CAD build for the part. Positions are in the model's coordinates, mm. A direction names the side the tool comes from. Round coordinates to 2 decimals unless told otherwise and drop trailing zeros. Order: outer loops, then holes, each group sorted by start corner. A loop starts at its lowest first (then second) coordinate and runs counter-clockwise, first axis right, second up. Notation, with made-up numbers: M 89,28.5 L 145,28.5 A17 cw 145,43.5 Z; hole C 27,73 d3. An arc over 180 degrees is marked long. Answer as a JSON object with one key per item and string values. Group by question number.
```python
from build123d import *

# Parameters (mm, degrees)
BOSS_EXTRUDE1_DEPTH = 36
FILLET2_R           = 8
SKETCH4_R           = 4
CUT_EXTRUDE2_DEPTH  = 32.38102997
SKETCH3_R           = 3
CUT_EXTRUDE3_DEPTH  = 12


with BuildPart() as part:
    # Sketch2 → Boss-Extrude1 (new body, symmetric)
    with BuildSketch(Plane(origin=(0, 0, 0), x_dir=(0, 0, -1), z_dir=(1, 0, 0))):
        Polygon((37.235479123, 0), (37.235479123, 12), (-34.764520877, 32.645667775), (-34.764520877, 0), align=None)
    extrude(amount=BOSS_EXTRUDE1_DEPTH, both=True)

    # Fillet2
    fillet2_edges = [part.edges().sort_by_distance(p)[0] for p in [
        (36, 6, -37.235479123),
        (-36, 6, -37.235479123),
        (-36, 16.322833887, 34.764520877),
        (36, 16.322833887, 34.764520877),
    ]]
    fillet(fillet2_edges, radius=FILLET2_R)

    # Sketch4 → Cut-Extrude2 (cut, through all)
    with BuildSketch(Plane(origin=(0, 20.954187427, -6.008516557), x_dir=(1, 0, 0), z_dir=(0, 0.961261696, -0.275637356))):
        with Locations((-23, 19.485391541)):
            Circle(SKETCH4_R)
    extrude(amount=-CUT_EXTRUDE2_DEPTH, mode=Mode.SUBTRACT)

    # Sketch3 → Cut-Extrude3 (cut)
    with BuildSketch(Plane(origin=(0, 20.954187427, -6.008516557), x_dir=(1, 0, 0), z_dir=(0, 0.961261696, -0.275637356))):
        with Locations((-20, -28.416167841)):
            Circle(SKETCH3_R)
        with Locations((-6, -28.416167841)):
            Circle(SKETCH3_R)
        with Locations((8, -28.416167841)):
            Circle(SKETCH3_R)
        with Locations((22, -28.416167841)):
            Circle(SKETCH3_R)
        with Locations((22, -14.416167841)):
            Circle(SKETCH3_R)
        with Locations((22, -0.416167841)):
            Circle(SKETCH3_R)
        with Locations((22, 13.583832159)):
            Circle(SKETCH3_R)
    extrude(amount=-CUT_EXTRUDE3_DEPTH, mode=Mode.SUBTRACT)


solid = part.part
```
Item 1: Drill centre lines: line 1 (X direction, y = 16.5, z = -4.5); line 2 (X direction, y = 2.5, z = -24); line 3 (Z direction, x = -25.5, y = 8). Where is each one in solid material? Low to high. Write a range as [from, to].
Item 2: Two-plate mould, pull along Y, no slides. Class faces 1 (the face through (0.5, 22.18, -1.74)), 2 (the face through (-33.594, 16.094, 32.483)), 3 (the face through (19, 19.2, 9.4)): +Y half, -Y half, draft (parallel to the pull), parting line (faces both ways), or undercut.
Item 3: Cut at A-A, the plane x = -8. Give the cut face in (y, z).
Item 4: Cut at B-B, the plane z = 29. Give the cut face in (x, y), and give its area (3 significant figures).
Item 5: Flat gauge pins, fed straight in: pin 1 Ø5 at (y, z) = (15.5, -29.5) entering from -X; pin 2 Ø10 at (x, z) = (-22.5, -27) entering from +Y. Where does each tip first touch, or does it go through?
Item 6: Cut at C-C, the plane x = 12. Give the cut face in (y, z).
Item 7: 3-axis set-ups, long thin cutter, end or side, ignore diameter. For faces 4 (the face through (7.96, 17.24, 24.57)), 5 (the face through (1, 0, -1)): which of +Z, -Z, +X, -X, +Y, -Y reach the whole face in a straight line?
Response values:
{
 "1": {"line 1": "[-36, 19.01], [24.99, 36]", "line 2": "[-36, -25.76], [-20.24, 36]", "line 3": "[-37.24, -25.81], [-19.32, 34.76]"},
 "2": {"face 1": "+Y half", "face 2": "draft", "face 3": "undercut"},
 "3": {"outline": "M 0,-37.24 L 12,-37.24 L 28.17,19.16 L 16.64,22.47 L 17.87,26.76 L 29.4,23.46 L 32.65,34.76 L 0,34.76 Z"},
 "4": {"outline": "M -35.68,0 L 35.68,0 L 35.68,30.99 L -35.68,30.99 Z", "area": "2,210 mm^2"},
 "5": {"pin 1": "x = -36", "pin 2": "y = 16.06"},
 "6": {"outline": "M 0,-37.24 L 12,-37.24 L 32.65,34.76 L 0,34.76 Z"},
 "7": {"face 4": "none", "face 5": "+Z, -Z, +X, -X, -Y"}
}
